Input: part model. Units: mm. Frame: model coordinates. Give positions to 0.01 mm unless a question says otherwise; leave off trailing zeros. Loops run counter-clockwise (first coordinate to the right, second up) from the corner with the lowest first, then second, coordinate; pieces in that order, holes last.
from build123d import *

# Parameters (mm, degrees)
EXTRUDE_4_DEPTH      = 100
EXTRUDE_4_DEPTH_BACK = 100
SKETCH_1_4_R         = 0.625


with BuildPart() as part:
    # Sketch 1_4 → Extrude 4 (new, two sides: drawn at the far end of the back side and taken through both)
    with BuildSketch(Plane(origin=(0, 0, 0), x_dir=(0, 0, -1), z_dir=(1, 0, 0)).offset(-EXTRUDE_4_DEPTH_BACK)):
        with BuildLine():
            Line((-4.5, 0), (0, 0))
            Line((0, 0), (4.5, 0))
            Line((4.5, 0), (4.5, 3.5))
            ThreePointArc((4.5, 3.5), (0, 8), (-4.5, 3.5))
            Line((-4.5, 3.5), (-4.5, 0))
        make_face()
        with Locations((-3.134058813, 1.75)):
            Circle(SKETCH_1_4_R, mode=Mode.SUBTRACT)
        with Locations((-1.224833948, 1.75)):
            Circle(SKETCH_1_4_R, mode=Mode.SUBTRACT)
        with Locations(Location((1.224833948, 1.75, 0), (0, 0, 180))):
            Circle(SKETCH_1_4_R, mode=Mode.SUBTRACT)
        with Locations(Location((3.134058813, 1.75, 0), (0, 0, 180))):
            Circle(SKETCH_1_4_R, mode=Mode.SUBTRACT)
        with BuildLine():
            Line((3.490727195, 3.5), (-3.490727195, 3.5))
            ThreePointArc((-3.490727195, 3.5), (0, 6.990727195), (3.490727195, 3.5))
        make_face(mode=Mode.SUBTRACT)
    extrude(amount=EXTRUDE_4_DEPTH + EXTRUDE_4_DEPTH_BACK)


solid = part.part
(1) Cut plane A-A (y = 5.5). Return the cut outline in (x, z), and give its area (3 significant figures).
Values follow:
outline: (-100, -4.03) - (100, -4.03) - (100, -2.86) - (-100, -2.86) - close; (-100, 2.86) - (100, 2.86) - (100, 4.03) - (-100, 4.03) - close
area: 468 mm2
(2) Mould query, pull axis Z, two halves, no side actions, for faces 1 (the flat face through (-1, 2, 4.5)), 2 (the flat face through (-1, 3.5, 0)), 3 (the flat face through (-1, 2, -4.5)). Classes: +Z half, -Z half, draft (parallel to the pull), parting line (faces both ways), or undercut.
Values follow:
face 1: +Z half
face 2: undercut
face 3: -Z half
(3) Ray query, probe 1 along Z at (x, y) = (-64.5, 1.5); probe 2 along Y at (x, z) = (41, -0.5); probe 3 along Y at (x, z) = (19, -1.5). Return the intervals inside material, ascending.
Values follow:
probe 1: z = -4.5 to -3.71, -2.56 to -1.8, -0.65 to 0.65, 1.8 to 2.56, 3.71 to 4.5
probe 2: y = 0 to 3.5, 6.95 to 7.97
probe 3: y = 0 to 1.19, 2.31 to 3.5, 6.65 to 7.74
(4) Cut plane B-B (x = -22.5). Return the cut outline in (y, z) (3 decimals), and give its area (3 significant figures).
Values follow:
outline: (0, -4.5) - (3.5, -4.5) arc R4.5 ccw to (3.5, 4.5) - (0, 4.5) - close; hole circle Ø1.25 at (1.75, -3.134); hole circle Ø1.25 at (1.75, -1.225); hole circle Ø1.25 at (1.75, 1.225); hole circle Ø1.25 at (1.75, 3.134); hole (3.5, -3.491) arc R3.491 ccw to (3.5, 3.491) - close
area: 39.3 mm2
(5) Pin query (flat end, axial travel): pin 1 Ø2 at (x, y) = (-67.5, 6.5) entering from -Z. Return the tip coordinate at first contact, or that it passes through.
Values follow:
pin 1: stops at z = -4.03
